Print and shaded views of the part. All mm, measured from the part's lowest x, y and z. Round coordinates to 2 decimals unless told otherwise and drop trailing zeros. Write each loop counter-clockwise with the first axis right and the second up, starting at its lowest first coordinate (ties: lowest second). Pieces come first, ordered by that corner, then holes. Notation, with made-up numbers: (-17.5, 83.25) - (13.5, 83.25) arc R16 cw to (13.5, 95.25) - close; hole circle Ø2 at (32.5, 77). An arc over 180 degrees is marked (long way). Answer as a JSON object with one key per item and string values. Group by question number.
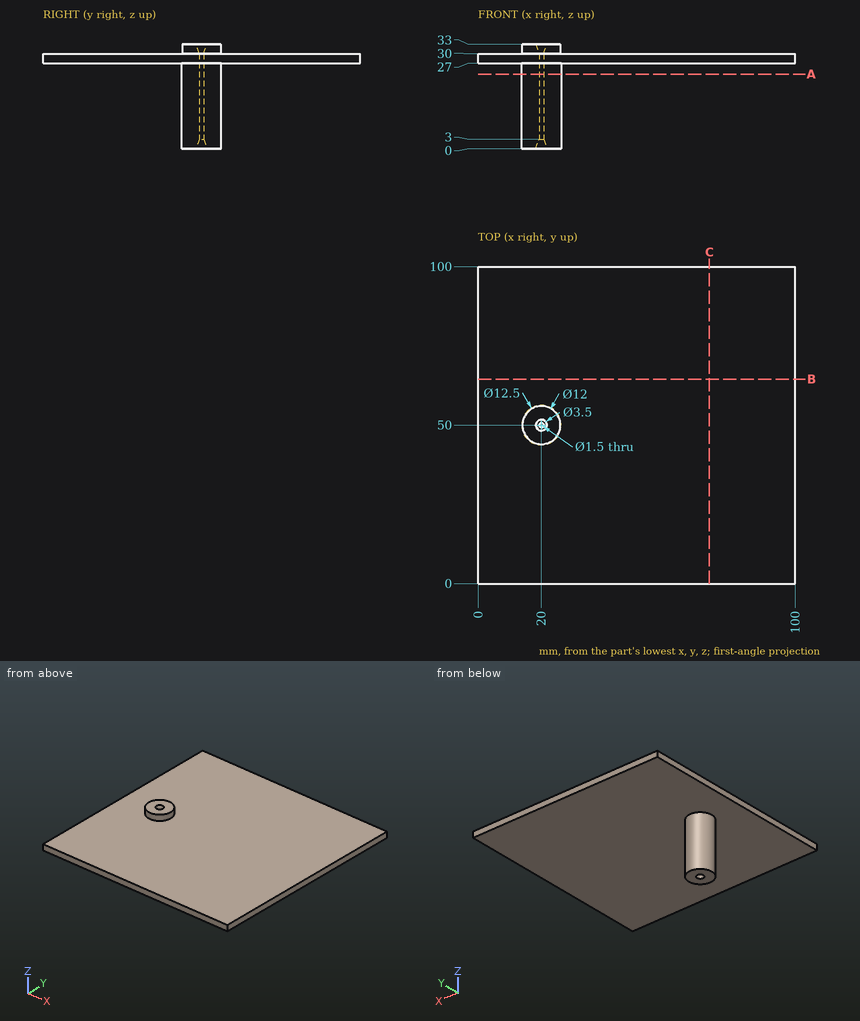
(1) Slice it at B-B (y = 64.5). Write the cut outline in (x, z), then the cut area to 3 significant figures.
(2) Slice it at A-A (z = 23.5). Write the cut outline in (x, y), then the cut area to 3 significant figures.
(3) Drill centre lines: line 1 (Y direction, x = 20, z = 15); line 2 (Z direction, x = 44.5, y = 44); line 3 (X direction, y = 47, z = 5.5). Where is each one in solid material? Low to high. Write a range as from..to.
(4) Flat gauge pins, fed straight in: pin 1 (1.4 mm diameter, centred on x = 20, y = 50, fed in from -Z); pin 2 (6 mm diameter, centred on x = 81, y = 80.5, fed in from -Z). Where does each tip first touch, or does it go through?
Answer:
{
 "1": {"outline": "(0, 27) - (100, 27) - (100, 30) - (0, 30) - close", "area": "300 mm²"},
 "2": {"outline": "circle Ø12.5 at (20, 50); hole circle Ø1.5 at (20, 50)", "area": "121 mm²"},
 "3": {"line 1": "43.75..49.25, 50.75..56.25", "line 2": "27..30", "line 3": "14.52..25.48"},
 "4": {"pin 1": "through", "pin 2": "z = 27"}
}
